Drawing for the job (mm, zero at the part's lowest x, y, z). Give positions to 0.01 mm unless a question says otherwise; leave off trailing zeros. Write each loop counter-clockwise with the first axis right and the second up, starting at its lowest first coordinate (ties: lowest second). Pieces come first, ordered by that corner, then holes.
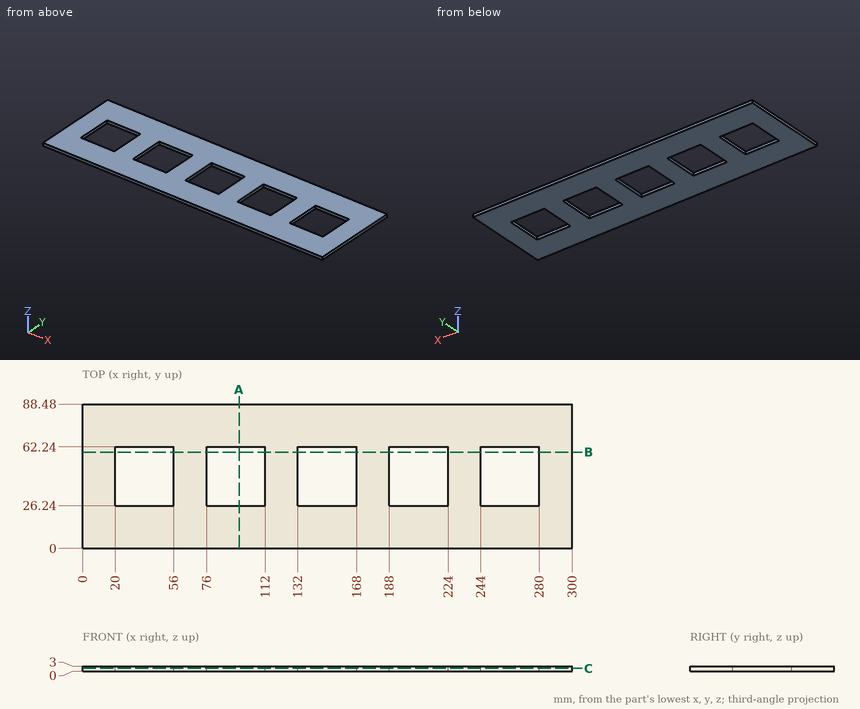
1. Pin check, flat tip, straight feed: P1, Ø1.5, axis at y = 41, z = 2.5, coming from the -X side. Stop position of the tip, or through.
Calculated:
P1: stops at x = 0
2. Probe probe 1 along X at (y, z) = (52.5, 0.25); probe 2 along Y at (x, z) = (97.5, 2.5). List the from-to ranges inside material, lowest first.
Calculated:
probe 1: x = 0 to 20, 56 to 76, 112 to 132, 168 to 188, 224 to 244, 280 to 300
probe 2: y = 0 to 26.24, 62.24 to 88.48
3. Slice it at C-C, the plane z = 1.85. Write the cut outline in (x, y).
Calculated:
outline: (0, 0) - (300, 0) - (300, 88.48) - (0, 88.48) - close; hole (20, 26.24) - (56, 26.24) - (56, 62.24) - (20, 62.24) - close; hole (76, 26.24) - (112, 26.24) - (112, 62.24) - (76, 62.24) - close; hole (132, 26.24) - (168, 26.24) - (168, 62.24) - (132, 62.24) - close; hole (188, 26.24) - (224, 26.24) - (224, 62.24) - (188, 62.24) - close; hole (244, 26.24) - (280, 26.24) - (280, 62.24) - (244, 62.24) - close
4. Slice it at B-B, the plane y = 59. Write the cut outline in (x, z), and give its area (3 significant figures).
Calculated:
outline: (0, 0) - (20, 0) - (20, 3) - (0, 3) - close; (56, 0) - (76, 0) - (76, 3) - (56, 3) - close; (112, 0) - (132, 0) - (132, 3) - (112, 3) - close; (168, 0) - (188, 0) - (188, 3) - (168, 3) - close; (224, 0) - (244, 0) - (244, 3) - (224, 3) - close; (280, 0) - (300, 0) - (300, 3) - (280, 3) - close
area: 360 mm2
5. Slice it at A-A, the plane x = 96. Write the cut outline in (y, z).
Calculated:
outline: (0, 0) - (26.24, 0) - (26.24, 3) - (0, 3) - close; (62.24, 0) - (88.48, 0) - (88.48, 3) - (62.24, 3) - close
